Autodesk Inventor part; units mm, degrees
ref_plane "YZ Plane" through (0, 0, 0) normal (1, 0, 0) x (0, 1, 0)
ref_plane "XZ Plane" through (0, 0, 0) normal (0, 1, 0) x (-1, 0, 0)
ref_plane "XY Plane" through (0, 0, 0) normal (0, 0, 1) x (1, 0, 0)
sketch "スケッチ4" plane through (0, 0, 0) normal (0, 0, 1) x (1, 0, 0)
  circle A0 centre (0, 0) radius 13.5
  circle A1 centre (0, 0) radius 23.5
  circle A2 centre (-14.5779, 11.3901) radius 5
  line L0 (13.5, 0) -> (78.5, 0)
  line L1 (78.5, 0) -> (78.5, 15)
  line L2 (78.5, 15) -> (13.5, 15)
  line L3 (13.5, 15) -> (13.5, 0)
  circle A3 centre (71, -7.5) radius 7.5
  line L4 (63.5, 0) -> (78.5, 0)
  line L5 (78.5, 0) -> (78.5, -7.5)
  line L6 (78.5, -7.5) -> (63.5, -7.5)
  line L7 (63.5, -7.5) -> (63.5, 0)
  point P0 (-10.6379, 8.3117)
  point P1 (78.5, 0)
  point P2 (18.0901, 15)
  point P3 (-18.5179, 14.4685)
  dimension "d15" = 27
  dimension "d19" = 15
  dimension "d16" = 47
  dimension "d17" = 65
  dimension "d18" = 15
extrude "押し出し3" add sketch "スケッチ4" along normal blind 6 contours L3 L2 A1 L0 | A0 A2 A1 L2 L3 | A2 | A1 L2 L1 L0 | L0 A3 L7 | L0 L5 A3 | A3 L6 | L6 A3
sketch "スケッチ5" plane through (0, 0, 0) normal (0, 0, -1) x (-1, 0, 0)
  line L0 (-78.5, -7.5) -> (-78.5, 15)
  line L1 (-63.5, 0) -> (-63.5, -7.5)
  line L2 (-78.5, 0) -> (-63.5, 0)
  line L3 (-63.5, 0) -> (-63.5, -7.5)
  line L4 (-63.5, -7.5) -> (-78.5, -7.5)
  line L5 (-78.5, -7.5) -> (-78.5, 0)
  circle A0 centre (-71, -7.5) radius 7.5
  point P0 (0, 0)
extrude "押し出し4" cut sketch "スケッチ5" against normal blind 3
sketch "スケッチ6" plane through (0, 0, 3) normal (0, 0, -1) x (-1, 0, 0)
  arc A0 (-78.5, -7.5) -> (-63.5, -7.5) centre (-71, -7.5) ccw
  point P0 (0, 0)
hole "穴2" at (71, -7.5, 3) direction (0, 0, 1) diameter 4.5 end through all
sketch "スケッチ7" plane through (18.0901, 15, 0) normal (0, 1, 0) x (1, 0, 0)
  line L0 (60.4099, -6) -> (0, -6)
  line L1 (-4.5901, 0) -> (60.4099, 0)
  line L2 (15, -6) -> (20, -6)
  line L3 (20, -6) -> (20, 0)
  line L4 (20, 0) -> (15, 0)
  line L5 (15, 0) -> (15, -6)
  line L6 (0, 0) -> (0, -6)
  point P0 (-18.0901, 0)
  dimension "d31" = 5
  dimension "d32" = 15
extrude "押し出し5" add sketch "スケッチ7" along normal blind 6 contours L0 L5 L1 L3
sketch "スケッチ8" plane through (38.0901, 15, 6) normal (1, 0, 0) x (0, 0, -1)
  line L0 (0, 0) -> (2, 0)
  line L1 (2, 0) -> (2, 2)
  line L2 (2, 2) -> (0, 2)
  line L3 (0, 2) -> (0, 0)
  point P0 (6, -15)
  dimension "d35" = 2
  dimension "d36" = 2
extrude "押し出し6" cut sketch "スケッチ8" against normal blind 6
properties part number "エアタンクペットボトル抑え２"
Input: part model. Units: mm. Frame: model coordinates. A direction names the side the tool comes from. Give positions to 0.01 mm unless a question says otherwise; leave off trailing zeros. Order: outer loops, then holes, each group sorted by start corner. A loop starts at its lowest first (then second) coordinate and runs counter-clockwise, first axis right, second up. Notation, with made-up numbers: (78.5, 33.25) - (120.5, 33.25) arc R15 cw to (120.5, 53.25) - close; hole circle Ø8 at (44.5, 89). An arc over 180 degrees is marked (long way). Use a Markdown table: item, result.
(1) Section query B-B (z = 4.9). Output: boundary loops of the cut face in (x, y), then the cut area to 3 significant figures.
Computed values:
| item | result |
|---|---|
| outline | (-18.52, 14.47) arc R5 ccw to (-10.64, 8.31) arc R13.5 cw to (13.5, 0) - (63.5, 0) - (63.5, -7.5) arc R7.5 ccw to (78.5, -7.5) - (78.5, 15) - (18.09, 15) arc R23.5 ccw to start; (33.09, 17) - (38.09, 17) - (38.09, 21) - (33.09, 21) - close; hole circle Ø4.5 at (71, -7.5) |
| area | 1,550 mm2 |
(2) Access query for faces 1 (the flat face through (36, 19, 6)), 2 (the flat face through (63.5, -4, 4)), 3 (the flat face through (36, 21, 3)), 4 (the flat face through (33.09, 18, 3)), 5 (the flat face through (36, 17, 5)). Directions: +Z, -Z, +X, -X, +Y, -Y. A direction counts if a zero-diameter tool reaches every point of the face in a straight line with its end or side. Return the directions, or none.
Computed values:
| item | result |
|---|---|
| face 1 | +Z, +X, -X, +Y, -Y |
| face 2 | +Z, -Z, -X, -Y |
| face 3 | +Z, -Z, +X, +Y |
| face 4 | +Z, -Z, +Y |
| face 5 | +Z, +X |
(3) Pin query (flat end, axial travel): pin 1 (2.5 mm diameter, centred on y = -3, z = 5, fed in from -X); pin 2 (1.8 mm diameter, centred on y = 18, z = 2, fed in from +X); pin 3 (2 mm diameter, centred on y = 2.5, z = 2, fed in from -X). Return the tip coordinate at first contact, or that it passes through.
Computed values:
| item | result |
|---|---|
| pin 1 | stops at x = 63.5 |
| pin 2 | stops at x = 38.09 |
| pin 3 | stops at x = 13.04 |
(4) Section query D-D (x = -6). Output: boundary loops of the cut face in (y, z), then the cut area to 3 significant figures.
Computed values:
| item | result |
|---|---|
| outline | (12.09, 0) - (22.72, 0) - (22.72, 6) - (12.09, 6) - close |
| area | 63.8 mm2 |
(5) Section query A-A (x = 71). Output: boundary loops of the cut face in (y, z).
Computed values:
| item | result |
|---|---|
| outline | (-15, 3) - (-9.75, 3) - (-9.75, 6) - (-15, 6) - close; (-5.25, 3) - (0, 3) - (0, 0) - (15, 0) - (15, 6) - (-5.25, 6) - close |
(6) Section query C-C (y = -4). Output: boundary loops of the cut face in (x, z), then the cut area to 3 significant figures.
Computed values:
| item | result |
|---|---|
| outline | (63.5, 3) - (78.5, 3) - (78.5, 6) - (63.5, 6) - close |
| area | 45.0 mm2 |
(7) Draft query along Y for faces 6 (the flat face through (69, -6, 3)), 7 (the cylindrical face through (4.17, 12.84, 2.96)), 8 (the flat face through (36, 16, 4)), 9 (the cylindrical face through (-17.569, 7.383, 2.958)). Return one class per face: released by +Y, released by -Y, zero draft, split by the parting line, or undercut.
Computed values:
| item | result |
|---|---|
| face 6 | zero draft |
| face 7 | released by -Y |
| face 8 | undercut |
| face 9 | split by the parting line |
(8) Line query: line 1 (X direction, y = -7.5, z = 5.1); line 2 (Y direction, x = 71, z = 5.15); line 3 (Y direction, x = 47, z = 2.75). Output: solid intervals per line, ascending. Write a range as from..to.
Computed values:
| item | result |
|---|---|
| line 1 | x = 63.5..68.75, 73.25..78.5 |
| line 2 | y = -15..-9.75, -5.25..15 |
| line 3 | y = 0..15 |
